Build history of the part. All positions in model axes, mm. A direction names the side the tool comes from. Give positions to 0.01 mm unless a question says otherwise; leave off trailing zeros. Write each loop counter-clockwise with the first axis right and the second up, starting at its lowest first coordinate (ties: lowest second). Pieces come first, ordered by that corner, then holes.
from build123d import *

# Parameters (mm, degrees)
F0_W     = 100
F0_H     = 100
F0_R     = 2.5
F1_DEPTH = 10
F2_R     = 2.5
F3_DEPTH = 25
F4_W     = 20
F4_H     = 20
F5_DEPTH = 5
F6_R     = 5
F7_DEPTH = 25
F8_R     = 5
F9_DEPTH = 5


with BuildPart() as f1:
    # F0 (on Top) → F1 (new body)
    with BuildSketch(Plane.XY):
        with Locations((50, 50)):
            Rectangle(F0_W, F0_H)
        with Locations((10, 50)):
            Circle(F0_R, mode=Mode.SUBTRACT)
    extrude(amount=F1_DEPTH)

    # F2 (on face) → F3 (join)
    with BuildSketch(Plane.XY.offset(10)):
        with Locations((72.9144066572, 20)):
            Circle(F2_R)
        with Locations((72.9144066572, 80)):
            Circle(F2_R)
    extrude(amount=F3_DEPTH)

    # F4 (on face) → F5 (join)
    with BuildSketch(Plane(origin=(0, 100, 0), x_dir=(-1, 0, 0), z_dir=(0, 1, 0))):
        with Locations((-45, 20)):
            Rectangle(F4_W, F4_H)
    extrude(amount=-F5_DEPTH)

    # F6 (on face) → F7 (cut)
    with BuildSketch(Plane(origin=(0, 100, 0), x_dir=(-1, 0, 0), z_dir=(0, 1, 0))):
        with Locations((-45, 20)):
            Circle(F6_R)
    extrude(amount=-F7_DEPTH, mode=Mode.SUBTRACT)

    # F8 (on face) → F9 (join)
    with BuildSketch(Plane.XZ):
        Polygon((95, 30), (95, 10), (100, 10), (115, 10), (115, 30), align=None)
        with Locations((105, 20)):
            Circle(F8_R, mode=Mode.SUBTRACT)
    extrude(amount=-F9_DEPTH)


solid = f1.part
1. Mould opens along Z. For faces 5 (the face through (49, 98, 17)), 6 (the face through (109.619, 2.465, 18.085)), 7 (the face through (70.417, 20.11, 22.325)), 8 (the face through (73, 20, 35)) say: pulls with the +Z half, pulls with the -Z half, needs draft (parallel to the pull), parting line crosses it, or undercut.
2. Drill centre lines: line 1 along Z through (x, y) = (105, 3); line 2 along Y through (x, z) = (10, 6); line 3 along Z through (x, y) = (45, 98). Where is each one in solid material? Low to high.
3. Saw through at A-A on x = 105. Give the cut face in (y, z).
4. Saw through at B-B on z = 20. Give the cut face in (x, y), plus the area to 3 significant figures.
5. 3-axis set-ups, long thin cutter, end or side, ignore diameter. For faces 1 (the face through (70.417, 80.11, 22.325)), 2 (the face through (103, 5, 25)), 3 (the face through (55, 98, 20)), 4 (the face through (107, 2, 10)): which of +Z, -Z, +X, -X, +Y, -Y reach the whole face in a straight line?
6. Saw through at C-C on y = 50. Give the cut face in (x, z), plus the area to 3 significant figures.
7. Drop flat-ended pins along their axis: pin 1 (10 mm diameter, centred on x = 106, z = 16.5, fed in from +Y); pin 2 (4 mm diameter, centred on x = 76.5, y = 72.5, fed in from +Z); pin 3 (2.5 mm diameter, centred on x = 111, y = 2, fed in from -Z); pin 4 (4.5 mm diameter, centred on x = 10, y = 50, fed in from +Z). Give the stop position or say it passes through.
8. Saw through at D-D on y = 80. Give the cut face in (x, z), plus the area to 4 significant figures.
Outcome:
1. face 5: undercut
1. face 6: undercut
1. face 7: needs draft
1. face 8: pulls with the +Z half
2. line 1: z = 10 to 15, 25 to 30
2. line 2: y = 0 to 47.5, 52.5 to 100
2. line 3: z = 0 to 15, 25 to 30
3. outline: (0, 10) - (5, 10) - (5, 15) - (0, 15) - close; (0, 25) - (5, 25) - (5, 30) - (0, 30) - close
4. outline: (35, 95) - (40, 95) - (40, 100) - (35, 100) - close; (50, 95) - (55, 95) - (55, 100) - (50, 100) - close; circle Ø5 at (72.91, 20); circle Ø5 at (72.91, 80); (95, 0) - (100, 0) - (100, 5) - (95, 5) - close; (110, 0) - (115, 0) - (115, 5) - (110, 5) - close
4. area: 139 mm2
5. face 1: +Z
5. face 2: +Z, +X, -X, +Y
5. face 3: +Z, +X, +Y, -Y
5. face 4: -Z, +X, +Y, -Y
6. outline: (0, 0) - (7.5, 0) - (7.5, 10) - (0, 10) - close; (12.5, 0) - (100, 0) - (100, 10) - (12.5, 10) - close
6. area: 950 mm2
7. pin 1: stops at y = 5
7. pin 2: stops at z = 10
7. pin 3: stops at z = 10
7. pin 4: passes through
8. outline: (0, 0) - (100, 0) - (100, 10) - (75.41, 10) - (75.41, 35) - (70.41, 35) - (70.41, 10) - (0, 10) - close
8. area: 1,125 mm2
